from build123d import *

# Parameters (mm, degrees)
SKETCH1_R              = 3.175
SKETCH1_R_2            = 10.499999955
SKETCH1_R_3            = 13.000000035
BOSS_EXTRUDE4_DEPTH    = 4.7625
F_10_CLEARANCE_HOLE3_D = 4.9784
SKETCH1_13_R           = 10.499999955
SKETCH1_13_R_2         = 9.000000034
SKETCH1_13_R_3         = 13.000000035
SKETCH1_13_R_4         = 10.750000026
BOSS_EXTRUDE5_DEPTH    = 0.79375


with BuildPart() as part:
    # Sketch1 → Boss-Extrude4 (new body)
    with BuildSketch(Plane.XY):
        with BuildLine():
            ThreePointArc((51.209487117, 68.380557282), (46.267175411, 96.444367544), (20.991271172, 109.60235205))
            ThreePointArc((20.991271172, 109.60235205), (10.314919955, 114.047741469), (5.487535559, 124.556895683))
            ThreePointArc((5.487535559, 124.556895683), (5.226909628, 127.186065068), (4.751663289, 129.785026101))
            ThreePointArc((4.751663289, 129.785026101), (-33.61376962, 154.665988281), (-58.191391536, 116.105526376))
            ThreePointArc((-58.191391536, 116.105526376), (-57.54504783, 113.543750167), (-56.690905362, 111.043570538))
            ThreePointArc((-56.690905362, 111.043570538), (-56.720922919, 99.478750551), (-64.589116092, 91.003050074))
            ThreePointArc((-64.589116092, 91.003050074), (-82.123671946, 68.541010041), (-74.972043993, 40.957353485))
            Line((-74.972043993, 40.957353485), (-22.715793489, -19.601472909))
            ThreePointArc((-22.715793489, -19.601472909), (6.372007721, -29.319320109), (28.80246523, -8.404939663))
            Line((28.80246523, -8.404939663), (51.209487117, 68.380557282))
        make_face()
        with BuildLine():
            Line((-53.146915005, 51.665951595), (-55.860861274, 53.313713912))
            ThreePointArc((-55.860861274, 53.313713912), (-59.272649919, 67.271181384), (-45.315182446, 70.682970029))
            Line((-45.315182446, 70.682970029), (-42.601236178, 69.035207713))
            ThreePointArc((-42.601236178, 69.035207713), (-39.189447533, 55.07774024), (-53.146915005, 51.665951595))
        make_face(mode=Mode.SUBTRACT)
        with Locations((-15.353270713, 70.644524994)):
            Circle(SKETCH1_R, mode=Mode.SUBTRACT)
        with Locations((-7.832512348, 36.039494433)):
            Circle(SKETCH1_R_2, mode=Mode.SUBTRACT)
        with BuildLine():
            Line((10.104747464, 80.489870832), (11.88996427, 83.11544238))
            ThreePointArc((11.88996427, 83.11544238), (26.004487005, 85.804577552), (28.693622177, 71.690054817))
            Line((28.693622177, 71.690054817), (26.90840537, 69.064483269))
            ThreePointArc((26.90840537, 69.064483269), (12.793882636, 66.375348097), (10.104747464, 80.489870832))
        make_face(mode=Mode.SUBTRACT)
        with BuildLine():
            Line((-36.027755896, 117.933191666), (-36.702042427, 121.035765223))
            ThreePointArc((-36.702042427, 121.035765223), (-28.931523946, 133.121717504), (-16.845571665, 125.351199024))
            Line((-16.845571665, 125.351199024), (-16.171285134, 122.248625467))
            ThreePointArc((-16.171285134, 122.248625467), (-23.941803614, 110.162673186), (-36.027755896, 117.933191666))
        make_face(mode=Mode.SUBTRACT)
        Circle(SKETCH1_R_3, mode=Mode.SUBTRACT)
    extrude(amount=-BOSS_EXTRUDE4_DEPTH)

    # #10 Clearance Hole3 (through all)
    with Locations(Plane.XY):
        with Locations((3.413684473, 96.21413667), (-43.040228891, 86.118244489), (-37.188807624, 83.578091132), (-32.235724588, 79.55833015), (-3.693450585, 85.761461384), (-0.855596504, 91.474437328), (36.598632596, 57.751177631), (41.153548262, 62.910968421), (44.277037033, 69.044035813), (26.566795152, 29.269907275), (-36.319050549, 15.602840887), (-57.267352023, 37.351155511), (-63.553004693, 40.154950839), (-68.940319132, 44.438353792), (-49.244623041, 111.062543152), (-51.540452576, 117.550983988), (-52.144800025, 124.407036926), (-1.402814067, 121.979927321), (-1.899275671, 128.33956849), (-4.087219361, 134.331597556)):
            Hole(F_10_CLEARANCE_HOLE3_D / 2)

    # Sketch1<13> → Boss-Extrude5 (add)
    # profile 1 of 2: a face of its own
    with BuildSketch(Plane.XY):
        with Locations((-7.832512348, 36.039494433)):
            Circle(SKETCH1_13_R)
        with Locations((-7.832512348, 36.039494433)):
            Circle(SKETCH1_13_R_2, mode=Mode.SUBTRACT)
    # profile 2 of 2: a face of its own
    with BuildSketch(Plane.XY):
        Circle(SKETCH1_13_R_3)
        Circle(SKETCH1_13_R_4, mode=Mode.SUBTRACT)
    extrude(amount=-BOSS_EXTRUDE5_DEPTH)


solid = part.part
Can you work these out from the model? Positions are in its coordinate system, mm. Coordinates: 2 decimals unless noted, no trailing zeros. Write each loop counter-clockwise with the first axis right and the second up, starting at its lowest first coordinate (ties: lowest second). Pieces come first, ordered by that corner, then holes.
Q1. Please list where these lines run through material, in increasing order: L1, parallel to Y at x = -10.5, z = -1; L2, parallel to X at y = 70.5, z = -3.55; L3, parallel to X at y = 37.5, z = -4.4.
Results found:
L1: y = -28.11 to -7.66, 7.66 to 25.88, 46.2 to 150.99
L2: x = -81.65 to -56.15, -45.01 to -18.52, -12.18 to 9.29, 27.88 to 42.26, 46.3 to 51.75
L3: x = -71.99 to -59.75, -54.78 to -18.23, 2.57 to 42.2
Q2. If we mould it in two halves opening along Y, with no side actions, what happens to faces 1 (the face through (-55.29, 35.84, -2.41)), 2 (the face through (-49.21, 11.1, -2.35)), 3 (the face through (5.23, 127.15, -2.35)), 4 (the face through (-49.054, 117.66, -2.415))? For each: +Y half, -Y half, draft (parallel to the pull), parting line (faces both ways), or undercut.
Results found:
face 1: undercut
face 2: -Y half
face 3: +Y half
face 4: undercut
Q3. Imagine slicing it at B-B, the plane y = 0. List the corners of the cut face in (x, z) for me, plus the area to 3 significant figures.
Results found:
outline: (-39.63, -4.76) - (-13, -4.76) - (-13, -0.79) - (-10.75, -0.79) - (-10.75, 0) - (-39.63, 0) - close; (10.75, -0.79) - (13, -0.79) - (13, -4.76) - (31.26, -4.76) - (31.26, 0) - (10.75, 0) - close
area: 217 mm2
Q4. Imagine slicing it at A-A, the plane x = 19. List the corners of the cut face in (y, z) for me, plus the area to 3 significant figures.
Results found:
outline: (-23.22, -4.76) - (64.63, -4.76) - (64.63, 0) - (-23.22, 0) - close; (87.48, -4.76) - (109.77, -4.76) - (109.77, 0) - (87.48, 0) - close
area: 525 mm2
Q5. Imagine slicing it at C-C, the plane z = -1.7. Count the separate pieces of the cut face and the enclosed holes in it, plus the area to 3 significant figures.
Results found:
separate pieces: 1
enclosed holes: 26
area: 13,700 mm2
Q6. For P1, Ø8, axis at x = -32.24, y = 79.56, coming from the +Z side; P2, Ø3, axis at x = -68.94, y = 44.44, coming from the +Z side; P3, Ø1.5, axis at y = 34, z = -2, coming from the -X side; P4, Ø1, axis at y = 81, z = -2.5, coming from the +X side, each with a flat end and sliding along its axis, tell me the tip position at first contact or that it passes through.
Results found:
P1: stops at z = 0
P2: passes through
P3: stops at x = -69.62
P4: stops at x = 52.35
